```python
from build123d import *

# Parameters (mm, degrees)
SKETCH_1_W      = 18
SKETCH_1_H      = 7
EXTRUDE_1_DEPTH = 1
SKETCH_3_R      = 1
EXTRUDE_2_DEPTH = 2
EXTRUDE_4_DEPTH = 0.5


with BuildPart() as part:
    # 草图1 → 凸台-拉伸1 (new body)
    with BuildSketch(Plane.XY):
        with Locations((-5.532426778, 1.915271967)):
            Rectangle(SKETCH_1_W, SKETCH_1_H)
    extrude(amount=EXTRUDE_1_DEPTH)

    # 草图3 → 凸台-拉伸2 (add)
    with BuildSketch(Plane.XY.offset(1)):
        with Locations((-11.532426778, 1.961868549)):
            Circle(SKETCH_3_R)
    extrude(amount=EXTRUDE_2_DEPTH)

    # 草图7 → 凸台-拉伸4 (add, symmetric)
    with BuildSketch(Plane(origin=(0.467573222, 0, 0), x_dir=(0, 0, -1), z_dir=(1, 0, 0))):
        Polygon((-2.5, 0.961868549), (-1, 0.961868549), (-1, 1.461868549), (-2, 1.461868549), (-2, 2.461868549), (-1, 2.461868549), (-1, 2.961868549), (-2.5, 2.961868549), align=None)
    extrude(amount=EXTRUDE_4_DEPTH, both=True)


solid = part.part
```
Check sheet for the modelled part. Datum: model origin and axes. Units: mm. A direction names the side the tool comes from. Coordinates: 2 decimals unless noted, no trailing zeros. Write each loop counter-clockwise with the first axis right and the second up, starting at its lowest first coordinate (ties: lowest second). Pieces come first, ordered by that corner, then holes. Notation, with made-up numbers: M -4,18 L 41,18 A27 ccw 41,37 Z; hole C 88.25,64.5 d1. An arc over 180 degrees is marked long. Write item = value, one per line. Start each with the question number.
1. Sectioned sample at B-B (y = 1.25). Record the cut outline in (x, z).
2. Thickness scan on probe 1 along Y at (x, z) = (0.5, 1.5); probe 2 along Z at (x, y) = (2.5, 0); probe 3 along X at (y, z) = (2.25, 2.15). Record the ranges inside material, lowest first.
3. Tool access check on faces 5 (the flat face through (0.5, 2.462, 1.5)), 6 (the flat face through (0.968, 2, 2.3)), 7 (the flat face through (0.5, 2.962, 1.7)), 8 (the flat face through (-5.7, 5.415, 0.5)), 9 (the flat face through (0.5, 0.962, 1.8)). Record the directions out of +Z, -Z, +X, -X, +Y, -Y that give a thin tool (end or side, any length) a straight path to the whole face; none if there is none.
4. Mould release check, pull along X, two halves, no side actions. Record for faces 1 (the flat face through (-0.032, 2, 2.3)), 2 (the flat face through (0.5, 2, 2.5)), 3 (the flat face through (-14.532, 1.9, 0.5)), 4 (the cylindrical face through (-10.6, 1.6, 2)): pulls with the +X half, pulls with the -X half, needs draft (parallel to the pull), parting line crosses it, or undercut.
5. Sectioned sample at D-D (z = 2.2). Record the cut outline in (x, y), then the cut area to 3 significant figures.
6. Sectioned sample at A-A (z = 1.35). Record the cut outline in (x, y), then the cut area to 3 significant figures.
7. Go/stop test with flat-tipped pins: pin 1 (2 mm diameter, centred on x = -3.5, y = 1, fed in from +Z); pin 2 (0.8 mm diameter, centred on y = 2, z = 2, fed in from -X); pin 3 (0.5 mm diameter, centred on x = 0.5, z = 2, fed in from -Y). Record where each tip stops, or that it passes through.
8. Sectioned sample at C-C (x = -13.5). Record the cut outline in (y, z).
The answers:
q1.outline = M -14.53,0 L 3.47,0 L 3.47,1 L 0.97,1 L 0.97,2.5 L -0.03,2.5 L -0.03,1 L -10.83,1 L -10.83,3 L -12.23,3 L -12.23,1 L -14.53,1 Z
q2.probe_1 = 0.96 to 1.46, 2.46 to 2.96
q2.probe_2 = 0 to 1
q2.probe_3 = -12.49 to -10.57, -0.03 to 0.97
q3.face_5 = +X
q3.face_6 = +Z, +X, +Y, -Y
q3.face_7 = +Z, +X, -X, +Y
q3.face_8 = +Z, -Z, +X, -X, +Y
q3.face_9 = +Z, +X, -X, -Y
q4.face_1 = undercut
q4.face_2 = needs draft
q4.face_3 = pulls with the -X half
q4.face_4 = undercut
q5.outline = C -11.53,1.96 d2; M -0.03,0.96 L 0.97,0.96 L 0.97,2.96 L -0.03,2.96 Z
q5.area = 5.14 mm²
q6.outline = C -11.53,1.96 d2; M -0.03,0.96 L 0.97,0.96 L 0.97,1.46 L -0.03,1.46 Z; M -0.03,2.46 L 0.97,2.46 L 0.97,2.96 L -0.03,2.96 Z
q6.area = 4.14 mm²
q7.pin_1 = 1
q7.pin_2 = -12.53
q7.pin_3 = 0.96
q8.outline = M -1.58,0 L 5.42,0 L 5.42,1 L -1.58,1 Z
